from build123d import *

# Parameters (mm, degrees)
F0_R     = 3.175
F1_DEPTH = 19.05
F2_R     = 6.35
F3_DEPTH = 4.445
F4_W     = 3.302
F4_H     = 26.5450086477
F5_DEPTH = 2.286
F6_R     = 1.27


with BuildPart() as f1:
    # F0 (on Top) → F1 (new body)
    with BuildSketch(Plane.XY):
        Circle(F0_R)
    extrude(amount=F1_DEPTH)

    # F2 (on face) → F3 (join)
    with BuildSketch(Plane(origin=(0, 0, 0), x_dir=(1, 0, 0), z_dir=(0, 0, -1))):
        Circle(F2_R)
    extrude(amount=F3_DEPTH)

    # F4 (on face) → F5 (cut)
    with BuildSketch(Plane(origin=(0, 0, -4.445), x_dir=(1, 0, 0), z_dir=(0, 0, -1))):
        Rectangle(F4_W, F4_H)
    extrude(amount=-F5_DEPTH, mode=Mode.SUBTRACT)

    # F6
    f6_edges = [f1.edges().sort_by_distance(p)[0] for p in [
        (-6.35, 0, -4.445),
        (5.040156, 3.862554, -4.445),
        (5.040156, -3.862554, -4.445),
    ]]
    fillet(f6_edges, radius=F6_R)


solid = f1.part
Check sheet for the modelled part. Datum: model origin and axes. Units: mm. A direction names the side the tool comes from. Give positions to 0.01 mm unless a question says otherwise; leave off trailing zeros. Loops run counter-clockwise (first coordinate to the right, second up) from the corner with the lowest first, then second, coordinate; pieces in that order, holes last. Notation, with made-up numbers: M -11.75,-38 L 6.25,-38 A30 cw 6.25,-12 Z; hole C 16.5,-15 d9. An arc over 180 degrees is marked long. Answer as a JSON object with one key per item and string values. Group by question number.
Q1. Cross-section at C-C on z = -1.25. Record the cut outline in (x, y), then the cut area to 3 significant figures.
Q2. Cross-section at B-B on x = 0. Record the cut outline in (y, z) (3 decimals), then the cut area to 3 significant figures.
Q3. Access from +Z, -Z, +X, -X, +Y, -Y to the whole of each face (thin tool, end or side, straight path). Record for faces 1 (the flat face through (3, 0, -4.445)), 2 (the flat face through (1.651, 0, -3)), 3 (the flat face through (-2, -3, 0)).
Q4. Go/stop test with flat-tipped pins: P1, Ø1.1, axis at y = 2, z = -3.5, coming from the -X side; P2, Ø1, axis at y = 1, z = 7.5, coming from the +X side; P3, Ø1.8, axis at y = -3, z = -3, coming from the +X side; P4, Ø3.5, axis at x = 0.5, y = 2.5, coming from the -Z side (3 decimals). Record where each tip stops, or that it passes through.
Q5. Release check for a two-part mould opening along X. For faces 4 (the flat face through (0, 0, -2.159)), 5 (the cylindrical face through (-0.69, -3.1, 9.39)), 6 (the flat face through (-3, 0, -4.445)) record: released by +X, released by -X, zero draft, split by the parting line, or undercut.
Q6. Cross-section at A-A on y = 0. Record the cut outline in (x, z) (3 decimals).
Q7. Material ranges on line 1 along Z through (x, y) = (4.25, 3); line 2 along X through (y, z) = (2.75, -3); line 3 along X through (y, z) = (-5.5, -0.25), recorded low to high. Write a range as [from, to].
Evaluation:
{
 "1": {"outline": "C 0,0 d12.7", "area": "127 mm2"},
 "2": {"outline": "M -6.35,-2.159 L 6.35,-2.159 L 6.35,0 L 3.175,0 L 3.175,19.05 L -3.175,19.05 L -3.175,0 L -6.35,0 Z", "area": "148 mm2"},
 "3": {"face 1": "-Z, +X, -X, +Y, -Y", "face 2": "-Z, +Y, -Y", "face 3": "+Z"},
 "4": {"P1": "stops at x = -6.17", "P2": "stops at x = 3.14", "P3": "stops at x = 5.99", "P4": "stops at z = -4.445"},
 "5": {"face 4": "undercut", "face 5": "split by the parting line", "face 6": "zero draft"},
 "6": {"outline": "M -6.35,-3.175 A1.27 ccw -5.08,-4.445 L -1.651,-4.445 L -1.651,-2.159 L 1.651,-2.159 L 1.651,-4.445 L 5.08,-4.445 A1.27 ccw 6.35,-3.175 L 6.35,0 L 3.175,0 L 3.175,19.05 L -3.175,19.05 L -3.175,0 L -6.35,0 Z"},
 "7": {"line 1": "z = [-4.44, 0]", "line 2": "x = [-5.72, -1.65], [1.65, 5.72]", "line 3": "x = [-3.17, 3.17]"}
}
